```python
from build123d import *

# Parameters (mm, degrees)
SKETCH1_W           = 176
SKETCH1_H           = 70
BOSS_EXTRUDE1_DEPTH = 30.5
SKETCH2_W           = 170
SKETCH2_H           = 64
CUT_EXTRUDE1_DEPTH  = 27.5
SKETCH3_W           = 176
SKETCH3_H           = 70
SKETCH3_W_2         = 173
SKETCH3_H_2         = 67
CUT_EXTRUDE2_DEPTH  = 5.5
FILLET1_R           = 2
SKETCH4_W           = 78
SKETCH4_H           = 31
SKETCH4_W_2         = 72
SKETCH4_H_2         = 25
BOSS_EXTRUDE2_DEPTH = 3
CUT_EXTRUDE3_REACH  = 5
SKETCH5_W           = 68
SKETCH5_H           = 15
CUT_EXTRUDE4_REACH  = 32.5
SKETCH6_R           = 1.75
CUT_EXTRUDE6_REACH  = 178


with BuildPart() as part:
    # Sketch1 → Boss-Extrude1 (new body)
    with BuildSketch(Plane(origin=(0, 0, 0), x_dir=(1, 0, 0), z_dir=(0, 1, 0))):
        Rectangle(SKETCH1_W, SKETCH1_H)
    extrude(amount=BOSS_EXTRUDE1_DEPTH)

    # Sketch2 → Cut-Extrude1 (cut)
    with BuildSketch(Plane.XZ):
        Rectangle(SKETCH2_W, SKETCH2_H)
    extrude(amount=-CUT_EXTRUDE1_DEPTH, mode=Mode.SUBTRACT)

    # Sketch3 → Cut-Extrude2 (cut)
    with BuildSketch(Plane.XZ):
        Rectangle(SKETCH3_W, SKETCH3_H)
        Rectangle(SKETCH3_W_2, SKETCH3_H_2, mode=Mode.SUBTRACT)
    extrude(amount=-CUT_EXTRUDE2_DEPTH, mode=Mode.SUBTRACT)

    # Fillet1
    fillet1_edges = [part.edges().sort_by_distance(p)[0] for p in [
        (88, 30.5, 0),
        (0, 30.5, -35),
        (-88, 30.5, 0),
        (-88, 18, -35),
        (88, 18, -35),
        (88, 18, 35),
        (-88, 18, 35),
        (0, 30.5, 35),
    ]]
    fillet(fillet1_edges, radius=FILLET1_R)

    # Sketch4 → Boss-Extrude2 (add)
    with BuildSketch(Plane.XZ.offset(-27.5)):
        with Locations((-31, 0.5)):
            Rectangle(SKETCH4_W, SKETCH4_H)
        with Locations((-31, 0.5)):
            Rectangle(SKETCH4_W_2, SKETCH4_H_2, mode=Mode.SUBTRACT)
    extrude(amount=BOSS_EXTRUDE2_DEPTH)

    # Sketch5 → Cut-Extrude3 (cut, up to next)
    with BuildSketch(Plane.XZ.offset(-27.5), mode=Mode.PRIVATE) as cut_extrude3_sk1:
        with Locations((-31, 0.5)):
            Rectangle(SKETCH5_W, SKETCH5_H)
    cut_extrude3_tool1 = extrude(cut_extrude3_sk1.sketch, amount=-CUT_EXTRUDE3_REACH, mode=Mode.PRIVATE) & part.part
    add(cut_extrude3_tool1.solids().sort_by_distance((-31, 27.5, 0.5))[0], mode=Mode.SUBTRACT)

    # Sketch6 → Cut-Extrude4 (cut, up to next)
    with BuildSketch(Plane(origin=(0, 30.5, 0), x_dir=(1, 0, 0), z_dir=(0, 1, 0)), mode=Mode.PRIVATE) as cut_extrude4_sk1:
        with Locations((-67.88, 14.57)):
            Circle(SKETCH6_R)
    cut_extrude4_tool1 = extrude(cut_extrude4_sk1.sketch, amount=-CUT_EXTRUDE4_REACH, mode=Mode.PRIVATE) & part.part
    add(cut_extrude4_tool1.solids().sort_by_distance((-67.88, 30.5, -14.57))[0], mode=Mode.SUBTRACT)
    # Sketch6 → Cut-Extrude4 (cut, up to next)
    with BuildSketch(Plane(origin=(0, 30.5, 0), x_dir=(1, 0, 0), z_dir=(0, 1, 0)), mode=Mode.PRIVATE) as cut_extrude4_sk2:
        with Locations((6.83, 14.57)):
            Circle(SKETCH6_R)
    cut_extrude4_tool2 = extrude(cut_extrude4_sk2.sketch, amount=-CUT_EXTRUDE4_REACH, mode=Mode.PRIVATE) & part.part
    add(cut_extrude4_tool2.solids().sort_by_distance((6.83, 30.5, -14.57))[0], mode=Mode.SUBTRACT)
    # Sketch6 → Cut-Extrude4 (cut, up to next)
    with BuildSketch(Plane(origin=(0, 30.5, 0), x_dir=(1, 0, 0), z_dir=(0, 1, 0)), mode=Mode.PRIVATE) as cut_extrude4_sk3:
        with Locations((6.83, -16.36)):
            Circle(SKETCH6_R)
    cut_extrude4_tool3 = extrude(cut_extrude4_sk3.sketch, amount=-CUT_EXTRUDE4_REACH, mode=Mode.PRIVATE) & part.part
    add(cut_extrude4_tool3.solids().sort_by_distance((6.83, 30.5, 16.36))[0], mode=Mode.SUBTRACT)
    # Sketch6 → Cut-Extrude4 (cut, up to next)
    with BuildSketch(Plane(origin=(0, 30.5, 0), x_dir=(1, 0, 0), z_dir=(0, 1, 0)), mode=Mode.PRIVATE) as cut_extrude4_sk4:
        with Locations((-67.88, -16.36)):
            Circle(SKETCH6_R)
    cut_extrude4_tool4 = extrude(cut_extrude4_sk4.sketch, amount=-CUT_EXTRUDE4_REACH, mode=Mode.PRIVATE) & part.part
    add(cut_extrude4_tool4.solids().sort_by_distance((-67.88, 30.5, 16.36))[0], mode=Mode.SUBTRACT)

    # Sketch8 → Cut-Extrude6 (cut, up to next)
    with BuildSketch(Plane(origin=(88, 0, 0), x_dir=(0, 0, -1), z_dir=(1, 0, 0)), mode=Mode.PRIVATE) as cut_extrude6_sk1:
        with BuildLine():
            Line((-22.5, 5.5), (-22.5, 0))
            Line((-22.5, 0), (-17.5, 0))
            Line((-17.5, 0), (-17.5, 5.5))
            ThreePointArc((-17.5, 5.5), (-20, 8), (-22.5, 5.5))
        make_face()
    cut_extrude6_tool1 = extrude(cut_extrude6_sk1.sketch, amount=-CUT_EXTRUDE6_REACH, mode=Mode.PRIVATE) & part.part
    add(cut_extrude6_tool1.solids().sort_by_distance((88, 3.752606, 20))[0], mode=Mode.SUBTRACT)


solid = part.part
```
Check sheet for the modelled part. Datum: model origin and axes. Units: mm. A direction names the side the tool comes from. Coordinates: 2 decimals unless noted, no trailing zeros. Order: outer loops, then holes, each group sorted by start corner. A loop starts at its lowest first (then second) coordinate and runs counter-clockwise, first axis right, second up. Notation, with made-up numbers: (-21.75, 76.25) -> (-12.75, 76.25) arc R16 ccw to (-12.75, 104.25) -> close; hole circle Ø4 at (0, 52.25). An arc over 180 degrees is marked (long way). Write item = value, one per line. Start each with the question number.
1) Access from +Z, -Z, +X, -X, +Y, -Y to the whole of each face (thin tool, end or side, straight path). Record for faces 4 (the flat face through (86.5, 3, -8)), 5 (the flat face through (85, 14, 0)), 6 (the flat face through (-31, 29, 8)).
2) Go/stop test with flat-tipped pins: P1, Ø5, axis at x = 5.5, z = -3, coming from the -Y side; P2, Ø6, axis at x = 10, y = 4, coming from the +Z side; P3, Ø1.5, axis at x = 11.5, z = 9, coming from the -Y side; P4, Ø0.9, axis at x = -18.5, y = 29.5, coming from the +Z side. Record where each tip stops, or that it passes through.
3) Cross-section at C-C (y = 14.5). Enter the section's corners in (x, z).
4) Mould release check, pull along Z, two halves, no side actions. Record for faces 1 (the flat face through (-1, 3, 33.5)), 2 (the flat face through (-1, 3, -33.5)), 3 (the flat face through (5, 26, 0)): +Z half, -Z half, draft (parallel to the pull), parting line (faces both ways), or undercut.
5) Material ranges on L1, parallel to Z at x = -67.88, y = 27.4; L2, parallel to X at y = 28, z = 16; L3, parallel to Z at x = 6.83, y = 28, recorded low to high.
6) Cross-section at A-A (x = -48). Enter the section's corners in (y, z), then the cut area to 3 significant figures.
7) Cross-section at B-B (z = 5). Enter the section's corners in (x, y), then the cut area to 3 significant figures.
8) Cross-section at D-D (x = 13). Enter the section's corners in (y, z).
Ans:
q1.face_4 = +Z, -Z, +X, -Y
q1.face_5 = -Y
q1.face_6 = +Y, -Y
q2.P1 = 24.5
q2.P2 = 35
q2.P3 = 27.5
q2.P4 = 34.92
q3.outline = (-88, -33) arc R2 ccw to (-86, -35) -> (86, -35) arc R2 ccw to (88, -33) -> (88, 33) arc R2 ccw to (86, 35) -> (-86, 35) arc R2 ccw to (-88, 33) -> close; hole (-85, -32) -> (85, -32) -> (85, 32) -> (-85, 32) -> close
q4.face_1 = +Z half
q4.face_2 = -Z half
q4.face_3 = undercut
q5.L1 = -35 to -32, -12.82 to 14.61, 32 to 35
q5.L2 = -88 to -69.59, -66.17 to 5.12, 8.54 to 88
q5.L3 = -35 to -16.32, -12.82 to 14.61, 18.11 to 35
q6.outline = (0, -33.5) -> (5.5, -33.5) -> (5.5, -35) -> (28.5, -35) arc R2 ccw to (30.5, -33) -> (30.5, -7) -> (27.5, -7) -> (27.5, -12) -> (24.5, -12) -> (24.5, -15) -> (27.5, -15) -> (27.5, -32) -> (0, -32) -> close; (0, 32) -> (27.5, 32) -> (27.5, 16) -> (24.5, 16) -> (24.5, 13) -> (27.5, 13) -> (27.5, 8) -> (30.5, 8) -> (30.5, 33) arc R2 ccw to (28.5, 35) -> (5.5, 35) -> (5.5, 33.5) -> (0, 33.5) -> close
q6.area = 330 mm²
q7.outline = (-88, 5.5) -> (-86.5, 5.5) -> (-86.5, 0) -> (-85, 0) -> (-85, 27.5) -> (-70, 27.5) -> (-70, 24.5) -> (-67, 24.5) -> (-67, 27.5) -> (-65, 27.5) -> (-65, 30.5) -> (-86, 30.5) arc R2 ccw to (-88, 28.5) -> close; (3, 27.5) -> (5, 27.5) -> (5, 24.5) -> (8, 24.5) -> (8, 27.5) -> (85, 27.5) -> (85, 0) -> (86.5, 0) -> (86.5, 5.5) -> (88, 5.5) -> (88, 28.5) arc R2 ccw to (86, 30.5) -> (3, 30.5) -> close
q7.area = 489 mm²
q8.outline = (0, -33.5) -> (5.5, -33.5) -> (5.5, -35) -> (28.5, -35) arc R2 ccw to (30.5, -33) -> (30.5, 33) arc R2 ccw to (28.5, 35) -> (5.5, 35) -> (5.5, 33.5) -> (0, 33.5) -> (0, 32) -> (27.5, 32) -> (27.5, -32) -> (0, -32) -> close
